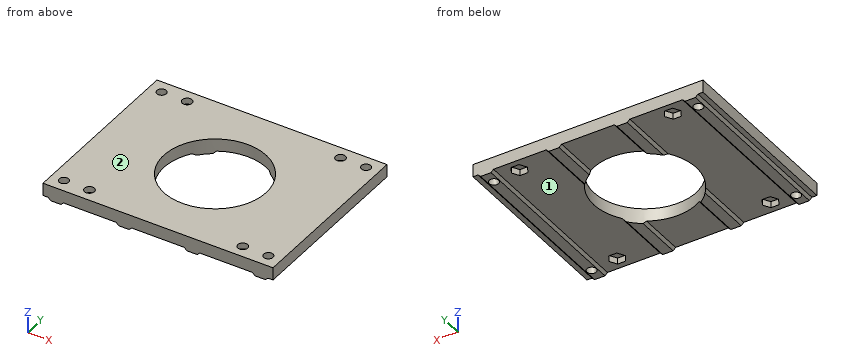
Autodesk Fusion 360 part; units mm, degrees
sketch "Sketch1" plane through (0, 0, 0) normal (0, 0, 1) x (1, 0, 0)
  line L0 (-45, 45) -> (45, 45) construction
  line L1 (45, 45) -> (45, -45) construction
  line L2 (45, -45) -> (-45, -45) construction
  line L3 (-45, -45) -> (-45, 45) construction
  line L4 (-45, 45) -> (45, -45) construction
  line L5 (45, 45) -> (-45, -45) construction
  circle A0 centre (-45, 45) radius 2.9
  circle A1 centre (45, 45) radius 2.9
  circle A2 centre (-45, -45) radius 2.9
  circle A3 centre (45, -45) radius 2.9
  line L6 (-60, 45) -> (60, 45) construction
  line L7 (60, 45) -> (60, -45) construction
  line L8 (60, -45) -> (-60, -45) construction
  line L9 (-60, -45) -> (-60, 45) construction
  line L10 (-60, 45) -> (60, -45) construction
  line L11 (60, 45) -> (-60, -45) construction
  circle A4 centre (-60, 45) radius 2.75
  circle A5 centre (60, 45) radius 2.75
  circle A6 centre (60, -45) radius 2.75
  circle A7 centre (-60, -45) radius 2.75
  line L12 (-67.5, 52.5) -> (67.5, 52.5)
  line L13 (67.5, 52.5) -> (67.5, -52.5)
  line L14 (67.5, -52.5) -> (-67.5, -52.5)
  line L15 (-67.5, -52.5) -> (-67.5, 52.5)
  line L16 (-67.5, 52.5) -> (67.5, -52.5) construction
  line L17 (67.5, 52.5) -> (-67.5, -52.5) construction
  circle A8 centre (0, 0) radius 30
  dimension "d1" = 90
  dimension "d2" = 90
  dimension "d3" = 5.8
  dimension "d4" = 5.8
  dimension "d5" = 5.8
  dimension "d6" = 5.8
  dimension "d7" = 120
  dimension "d8" = 90
  dimension "d9" = 5.5
  dimension "d10" = 5.5
  dimension "d11" = 5.5
  dimension "d12" = 5.5
  dimension "d13" = 135
  dimension "d14" = 105
  dimension "d27" = 60
extrude "Extrude1" add sketch "Sketch1" along normal blind 3.6
sketch "Sketch2" plane through (0, 0, 0) normal (0, 0, -1) x (1, 0, 0)
  circle A0 centre (-45, -45) radius 2.9
  circle A1 centre (-60, -45) radius 2.75
  circle A2 centre (60, -45) radius 2.75
  circle A3 centre (-60, 45) radius 2.75
  circle A4 centre (45, -45) radius 2.9
  circle A5 centre (-45, 45) radius 2.9
  circle A6 centre (45, 45) radius 2.9
  circle A7 centre (60, 45) radius 2.75
  line L0 (67.5, 52.5) -> (-67.5, 52.5)
  line L1 (-67.5, 52.5) -> (-67.5, -52.5)
  line L2 (-67.5, -52.5) -> (67.5, -52.5)
  line L3 (67.5, -52.5) -> (67.5, 52.5)
  line L4 (-67.5, 52.5) -> (67.5, 52.5)
  line L5 (67.5, 52.5) -> (67.5, -52.5)
  line L6 (67.5, -52.5) -> (-67.5, -52.5)
  line L7 (-67.5, -52.5) -> (-67.5, 52.5)
  line L8 (-67.5, 52.5) -> (67.5, -52.5) construction
  line L9 (67.5, 52.5) -> (-67.5, -52.5) construction
  circle A8 centre (0, 0) radius 30
  dimension "d17" = 135
  dimension "d18" = 105
extrude "Extrude2" add sketch "Sketch2" along normal blind 0.2 contours A0 | A4 | A5 | A6 | L0 L1 L2 L3 L4 L5 L6 L7
sketch "Sketch3" plane through (0, 0, -0.2) normal (0, 0, -1) x (1, 0, 0)
  circle A0 centre (-60, -45) radius 2.75
  circle A1 centre (60, -45) radius 2.75
  circle A2 centre (-60, 45) radius 2.75
  circle A3 centre (60, 45) radius 2.75
  line L0 (-67.5, -52.5) -> (67.5, -52.5)
  line L1 (67.5, -52.5) -> (67.5, 52.5)
  line L2 (67.5, 52.5) -> (-67.5, 52.5)
  line L3 (-67.5, 52.5) -> (-67.5, -52.5)
  line L4 (-42.6329, 40.9) -> (-40.2657, 45)
  line L5 (-40.2657, 45) -> (-42.6329, 49.1)
  line L6 (-42.6329, 49.1) -> (-47.3671, 49.1)
  line L7 (-47.3671, 49.1) -> (-49.7343, 45)
  line L8 (-49.7343, 45) -> (-47.3671, 40.9)
  line L9 (-47.3671, 40.9) -> (-42.6329, 40.9)
  line L10 (-47.3671, -40.9) -> (-49.7343, -45)
  line L11 (-49.7343, -45) -> (-47.3671, -49.1)
  line L12 (-47.3671, -49.1) -> (-42.6329, -49.1)
  line L13 (-42.6329, -49.1) -> (-40.2657, -45)
  line L14 (-40.2657, -45) -> (-42.6329, -40.9)
  line L15 (-42.6329, -40.9) -> (-47.3671, -40.9)
  line L16 (47.3671, 40.9) -> (49.7343, 45)
  line L17 (49.7343, 45) -> (47.3671, 49.1)
  line L18 (47.3671, 49.1) -> (42.6329, 49.1)
  line L19 (42.6329, 49.1) -> (40.2657, 45)
  line L20 (40.2657, 45) -> (42.6329, 40.9)
  line L21 (42.6329, 40.9) -> (47.3671, 40.9)
  line L22 (42.6329, -40.9) -> (40.2657, -45)
  line L23 (40.2657, -45) -> (42.6329, -49.1)
  line L24 (42.6329, -49.1) -> (47.3671, -49.1)
  line L25 (47.3671, -49.1) -> (49.7343, -45)
  line L26 (49.7343, -45) -> (47.3671, -40.9)
  line L27 (47.3671, -40.9) -> (42.6329, -40.9)
  circle A4 centre (0, 0) radius 30
  point P0 (-45, 45)
  point P1 (-45, -45)
  point P2 (45, 45)
  point P3 (45, -45)
  dimension "d21" = 4.1
  dimension "d22" = 4.1
  dimension "d23" = 4.1
  dimension "d24" = 4.1
extrude "Extrude3" add sketch "Sketch3" along normal blind 3.6
sketch "Sketch4" plane through (-67.5, 0, 0) normal (-1, 0, 0) x (0, -1, 0)
  line L0 (52.5, -3.8) -> (52.5, 3.6)
  line L1 (52.5, 3.6) -> (-52.5, 3.6)
  line L2 (-52.5, 3.6) -> (-52.5, -3.8)
  line L3 (-52.5, -3.8) -> (52.5, -3.8)
  line L4 (-3.0507, 8.6121) -> (-4.3315, 9.8929)
  line L5 (-4.8314, 10.1) -> (-3.6911, 10.1) construction
  line L6 (-4.8314, 10.1) -> (-4.5386, 10.1) construction
  line L7 (4.3315, 9.8929) -> (3.0507, 8.6121)
  line L8 (-3.0507, 8.6121) -> (3.0507, 8.6121)
  line L9 (4.8314, 10.1) -> (4.5386, 10.1) construction
  line L10 (4.3315, 9.8929) -> (4.5386, 10.1)
  line L11 (-4.3315, 9.8929) -> (-4.5386, 10.1)
  line L12 (-52.5, -0.1) -> (-45, -0.1) construction
  line L13 (52.5, -0.1) -> (45, -0.1) construction
sketch "Sketch5" plane through (0, -52.5, 0) normal (0, -1, 0) x (1, 0, 0)
  line L0 (67.5, -3.8) -> (67.5, 3.6)
  line L1 (67.5, 3.6) -> (-67.5, 3.6)
  line L2 (-67.5, 3.6) -> (-67.5, -3.8)
  line L3 (-67.5, -3.8) -> (67.5, -3.8)
  line L4 (15.1684, -3.7997) -> (16.3088, -3.7997) construction
  line L5 (15.6684, -4.0068) -> (15.4613, -3.7997)
  line L6 (15.1684, -3.7997) -> (15.4613, -3.7997) construction
  line L7 (24.8313, -3.7997) -> (24.5385, -3.7997) construction
  line L8 (16.9492, -5.2876) -> (23.0506, -5.2876)
  line L9 (24.3314, -4.0068) -> (24.5385, -3.7997)
  line L10 (24.3314, -4.0068) -> (23.0506, -5.2876)
  line L11 (16.9492, -5.2876) -> (15.6684, -4.0068)
  line L12 (-67.5, -0.1) -> (-60, -0.1) construction
  line L13 (-60, -0.1) -> (60, -0.1) construction
  line L14 (60, -0.1) -> (67.5, -0.1) construction
  line L15 (-60, -0.1) -> (-20, -0.1) construction
  line L16 (60, -0.1) -> (20, -0.1) construction
  line L17 (-20, -0.1) -> (-20, 10.5) construction
  line L18 (16.9492, -5.2876) -> (19.9999, -5.2876) construction
  line L19 (-23.0508, -5.2876) -> (-20.0001, -5.2876) construction
  line L20 (-15.6686, -4.0068) -> (-15.4615, -3.7997)
  line L21 (-24.8316, -3.7997) -> (-23.6912, -3.7997) construction
  line L22 (-23.0508, -5.2876) -> (-16.9494, -5.2876)
  line L23 (-15.6686, -4.0068) -> (-16.9494, -5.2876)
  line L24 (-23.0508, -5.2876) -> (-24.3316, -4.0068)
  line L25 (-24.8316, -3.7997) -> (-24.5387, -3.7997) construction
  line L26 (-24.3316, -4.0068) -> (-24.5387, -3.7997)
  line L27 (-15.1687, -3.7997) -> (-15.4615, -3.7997) construction
  line L28 (64.8313, -3.7997) -> (64.5385, -3.7997) construction
  line L29 (56.9492, -5.2876) -> (59.9999, -5.2876) construction
  line L30 (64.3314, -4.0068) -> (63.0506, -5.2876)
  line L31 (55.6684, -4.0068) -> (55.4613, -3.7997)
  line L32 (56.9492, -5.2876) -> (55.6684, -4.0068)
  line L33 (55.1684, -3.7997) -> (55.4613, -3.7997) construction
  line L34 (56.9492, -5.2876) -> (63.0506, -5.2876)
  line L35 (64.3314, -4.0068) -> (64.5385, -3.7997)
  line L36 (55.1684, -3.7997) -> (56.3088, -3.7997) construction
  line L37 (-63.0508, -5.2876) -> (-64.3316, -4.0068)
  line L38 (-63.0508, -5.2876) -> (-60.0001, -5.2876) construction
  line L39 (-64.3316, -4.0068) -> (-64.5387, -3.7997)
  line L40 (-55.6686, -4.0068) -> (-56.9494, -5.2876)
  line L41 (-63.0508, -5.2876) -> (-56.9494, -5.2876)
  line L42 (-55.6686, -4.0068) -> (-55.4615, -3.7997)
  line L43 (-64.8316, -3.7997) -> (-64.5387, -3.7997) construction
  line L44 (-55.1687, -3.7997) -> (-55.4615, -3.7997) construction
  line L45 (-64.8316, -3.7997) -> (-63.6912, -3.7997) construction
extrude "Extrude4" add sketch "Sketch5" against normal blind 105 contours L3 L30 L31 L32 L34 L35 | L3 L5 L8 L9 L10 L11 | L3 L37 L39 L40 L41 L42 | L3 L20 L22 L23 L24 L26
extrude "Extrude5" cut sketch "Sketch3" along normal blind 6 contours A0 | A1 | A2 | A3 | A4
Geometry: final body of the model. Coordinates: model frame, mm. Face numbers are marked on the shaded views. Round coordinates to 2 decimals unless told otherwise and drop trailing zeros. Loops run counter-clockwise (first coordinate to the right, second up) from the corner with the lowest first, then second, coordinate; pieces in that order, holes last. Notation, with made-up numbers: (-8, 36) -> (45, 36) arc R12 ccw to (45, 49) -> close; hole circle Ø10 at (-30.5, 37.25). An arc over 180 degrees is marked (long way). Use one line per item in the form item = value. Start each with the question number.
1) Section B-B on z = 2. Give the number of separate pieces and of enclosed holes in the cut face, then the cut area to 3 significant figures.
2) First-contact query: P1, Ø9, axis at x = 46, y = -44, coming from the -Z side; P2, Ø4.5, axis at x = -45, y = 45, coming from the -Z side; P3, Ø4.5, axis at x = 60, y = 45, coming from the +Z side (3 decimals). Flat tips, straight axial feed; report the tip coordinate or a pass-through.
3) Section C-C on x = 60. Output: boundary loops of the cut face in (y, z), then the cut area to 3 significant figures.
4) Draft query along X for the marked faces 1 and 2. Return one class per face: released by +X, released by -X, zero draft, split by the parting line, or undercut.
5) Section A-A on y = 0. Output: boundary loops of the cut face in (x, z).
6) Line query: L1, parallel to Y at x = 45, z = 1.05; L2, parallel to Y at x = 60, z = -2; L3, parallel to X at y = -22, z = -1.25. Output: solid intervals per line, ascending.
7) Section D-D on x = 0. Output: boundary loops of the cut face in (y, z).
Response:
q1.separate_pieces = 1
q1.enclosed_holes = 9
q1.area = 11,100 mm^2
q2.P1 = -3.8
q2.P2 = -0.2
q2.P3 = through
q3.outline = (-52.5, -5.29) -> (-47.75, -5.29) -> (-47.75, 3.6) -> (-52.5, 3.6) -> close; (-42.25, -5.29) -> (42.25, -5.29) -> (42.25, 3.6) -> (-42.25, 3.6) -> close; (47.75, -5.29) -> (52.5, -5.29) -> (52.5, 3.6) -> (47.75, 3.6) -> close
q3.area = 835 mm^2
q4.face_1 = undercut
q4.face_2 = zero draft
q5.outline = (-67.5, -3.8) -> (-64.54, -3.8) -> (-63.05, -5.29) -> (-56.95, -5.29) -> (-55.46, -3.8) -> (-30, -3.8) -> (-30, 3.6) -> (-67.5, 3.6) -> close; (30, -3.8) -> (55.46, -3.8) -> (56.95, -5.29) -> (63.05, -5.29) -> (64.54, -3.8) -> (67.5, -3.8) -> (67.5, 3.6) -> (30, 3.6) -> close
q6.L1 = -52.5 to -47.9, -42.1 to 42.1, 47.9 to 52.5
q6.L2 = -52.5 to -47.75, -42.25 to 42.25, 47.75 to 52.5
q6.L3 = -67.5 to -20.4, 20.4 to 67.5
q7.outline = (-52.5, -3.8) -> (-30, -3.8) -> (-30, 3.6) -> (-52.5, 3.6) -> close; (30, -3.8) -> (52.5, -3.8) -> (52.5, 3.6) -> (30, 3.6) -> close
